Verification items for the finished model (mm, model axes). A direction names the side the tool comes from. Coordinates: 2 decimals unless noted, no trailing zeros. Write each loop counter-clockwise with the first axis right and the second up, starting at its lowest first coordinate (ties: lowest second). Pieces come first, ordered by that corner, then holes. Notation, with made-up numbers: (-14, 12.25) -> (44, 12.25) arc R27 ccw to (44, 51.25) -> close; hole circle Ø8 at (66, 1.5). An arc over 180 degrees is marked (long way). Write item = value, one per line. Start each with the question number.
(1) Section check B-B (y = -96.52). Record the cut outline in (x, z) (3 decimals), plus the area to 3 significant figures.
(2) Set-up check for faces 1 (the face through (-19, -469.9, -5)), 2 (the face through (180, 0, -5)), 3 (the face through (-19, -571.5, -5)), 4 (the face through (-11.6, -18.8, -4.9)), 5 (the face through (350.168, -500.631, -3.863)): record each of +Z, -Z, +X, -X, +Y, -Y from which the full face is reachable in a straight line by a thin tool's end or side.
(3) Gauge pin test, flat ends, axial feed: pin 1 Ø12 at (x, y) = (137, -469.5) entering from -Z; pin 2 Ø2 at (y, z) = (-77, -7) entering from -X. Record the tip position at first contact, or that the pin passes through.
(4) Section check D-D (y = -319). Record the cut outline in (x, z).
(5) Section check A-A (x = 342.9). Record the cut outline in (y, z), plus the area to 3 significant figures.
(6) Material ranges on probe 1 along Y at (x, z) = (342.9, -4.5); probe 2 along Z at (x, y) = (94.5, -353); probe 3 along X at (y, z) = (-174, -1.5), recorded low to high. Write a range as [from, to].
(7) Mould release check, pull along X, two halves, no side actions. Record for faces 6 (the face through (-19, -546.1, -5)), 7 (the face through (349.94, -99.44, -3.86)), 8 (the face through (-11.6, -126.8, -4.9)): released by +X, released by -X, zero draft, split by the parting line, or undercut.
(8) Section check C-C (x = 105.5). Record the cut outline in (y, z), plus the area to 3 significant figures.
```python
from build123d import *

# Parameters (mm, degrees)
BOSS_EXTRUDE1_DEPTH     = 609.6
SHELL1_T                = -7.62
SKETCH3_W               = 28.861952205
SKETCH3_H               = 274.814581436
CUT_EXTRUDE2_DEPTH      = 609.6
SKETCH4_W               = 397.1798
SKETCH4_H               = 244.7798
CUT_EXTRUDE3_DEPTH      = 609.6
SKETCH5_W               = 397.1798
SKETCH5_H               = 7.62
CUT_EXTRUDE4_DEPTH      = 609.6
BOSS_EXTRUDE4_START     = 25.4
BOSS_EXTRUDE4_DEPTH     = 25.4
LPATTERN2_COUNT         = 3
LPATTERN2_PITCH         = 50.8
LPATTERN3_COUNT         = 2
LPATTERN3_PITCH         = 508
LPATTERN6_COUNT         = 2
LPATTERN6_PITCH         = 457.2
LPATTERN7_COUNT         = 2
LPATTERN7_PITCH         = 406.4
CUT_EXTRUDE5_DEPTH      = 660.835961681
CUT_EXTRUDE5_DEPTH_BACK = 660.835961681
SKETCH11_R              = 4.445
CUT_EXTRUDE6_DEPTH      = 660.835961681
CUT_EXTRUDE6_DEPTH_BACK = 660.835961681
CUT_EXTRUDE7_DEPTH      = 681.722733812
CUT_EXTRUDE7_DEPTH_BACK = 681.722733812
CUT_EXTRUDE8_DEPTH      = 713.602768959
CUT_EXTRUDE8_DEPTH_BACK = 713.602768959
SKETCH16_R              = 7.62


with BuildPart() as part:
    # Sketch1 → Boss-Extrude1 (new body)
    with BuildSketch(Plane(origin=(0, 0, 0), x_dir=(1, 0, 0), z_dir=(0, 1, 0))):
        with BuildLine():
            Line((0, 0), (381, 0))
            ThreePointArc((381, 0), (392.440846298, 4.738953702), (397.1798, 16.1798))
            Line((397.1798, 16.1798), (397.1798, 244.7798))
            ThreePointArc((397.1798, 244.7798), (392.440846298, 256.220646298), (381, 260.9596))
            Line((381, 260.9596), (0, 260.9596))
            ThreePointArc((0, 260.9596), (-11.440846298, 256.220646298), (-16.1798, 244.7798))
            Line((-16.1798, 244.7798), (-16.1798, 16.1798))
            ThreePointArc((-16.1798, 16.1798), (-11.440846298, 4.738953702), (0, 0))
        make_face()
    extrude(amount=-BOSS_EXTRUDE1_DEPTH)

    # Shell1
    shell1_openings = [part.faces().sort_by_distance(p)[0] for p in [
        (190.5, 0, -130.4798),
    ]]
    offset(amount=SHELL1_T, openings=shell1_openings, kind=Kind.INTERSECTION)

    # Sketch3 → Cut-Extrude2 (cut)
    with BuildSketch(Plane(origin=(0, 0, 0), x_dir=(1, 0, 0), z_dir=(0, 1, 0))):
        with Locations((395.430976103, 137.407290718)):
            Rectangle(SKETCH3_W, SKETCH3_H)
    extrude(amount=-CUT_EXTRUDE2_DEPTH, mode=Mode.SUBTRACT)

    # Sketch4 → Cut-Extrude3 (cut)
    with BuildSketch(Plane(origin=(0, 0, 0), x_dir=(1, 0, 0), z_dir=(0, 1, 0))):
        with Locations((182.4101, 138.5697)):
            Rectangle(SKETCH4_W, SKETCH4_H)
    extrude(amount=-CUT_EXTRUDE3_DEPTH, mode=Mode.SUBTRACT)

    # Sketch5 → Cut-Extrude4 (cut)
    with BuildSketch(Plane(origin=(0, 0, -16.1798), x_dir=(-1, 0, 0), z_dir=(0, 0, -1))):
        with Locations((-182.4101, -605.79)):
            Rectangle(SKETCH5_W, SKETCH5_H)
    extrude(amount=-CUT_EXTRUDE4_DEPTH, mode=Mode.SUBTRACT)

    # Sketch8 → Boss-Extrude4 (add)
    with BuildSketch(Plane(origin=(0, -63.5, 0), x_dir=(1, 0, 0), z_dir=(0, 1, 0)).offset(BOSS_EXTRUDE4_START)):
        with BuildLine():
            Line((-16.1798, 16.1798), (-31.4198, 16.1798))
            Line((-31.4198, 16.1798), (-31.4198, 3.2512))
            ThreePointArc((-31.4198, 3.2512), (-30.467545567, 0.952254433), (-28.1686, 0))
            Line((-28.1686, 0), (0, 0))
            ThreePointArc((0, 0), (-11.440846298, 4.738953702), (-16.1798, 16.1798))
        make_face()
    boss_extrude4 = extrude(amount=-BOSS_EXTRUDE4_DEPTH)

    # LPattern2: Boss-Extrude4 ×3
    with Locations(*[(0, -i * LPATTERN2_PITCH, 0) for i in range(1, LPATTERN2_COUNT)]):
        add(boss_extrude4)

    # LPattern3: Boss-Extrude4 ×2
    with Locations(*[(0, -i * LPATTERN3_PITCH, 0) for i in range(1, LPATTERN3_COUNT)]):
        add(boss_extrude4)

    # LPattern6: Boss-Extrude4 ×2
    with Locations(*[(0, -i * LPATTERN6_PITCH, 0) for i in range(1, LPATTERN6_COUNT)]):
        add(boss_extrude4)

    # LPattern7: Boss-Extrude4 ×2
    with Locations(*[(0, -i * LPATTERN7_PITCH, 0) for i in range(1, LPATTERN7_COUNT)]):
        add(boss_extrude4)

    # Sketch11 → Cut-Extrude5 (cut, two sides: drawn at the far end of the back side and taken through both)
    with BuildSketch(Plane(origin=(0, -63.5, 0), x_dir=(1, 0, 0), z_dir=(0, 1, 0)).offset(-CUT_EXTRUDE5_DEPTH_BACK)):
        with Locations(Location((-22.7838, 8.5598, 0), (0, 0, 270))):
            Circle(SKETCH11_R)
    extrude(amount=CUT_EXTRUDE5_DEPTH + CUT_EXTRUDE5_DEPTH_BACK, mode=Mode.SUBTRACT)

    # Sketch14 → Cut-Extrude6 (cut, two sides: drawn at the far end of the back side and taken through both)
    with BuildSketch(Plane(origin=(0, -63.5, 0), x_dir=(1, 0, 0), z_dir=(0, 1, 0)).offset(-CUT_EXTRUDE6_DEPTH_BACK)):
        with BuildLine():
            Line((-23.2901518, 16.1798), (-23.2901518, 22.367061587))
            Line((-23.2901518, 22.367061587), (-43.448334217, 22.367061587))
            Line((-43.448334217, 22.367061587), (-43.448334217, 8.0501518))
            Line((-43.448334217, 8.0501518), (-31.4198, 8.0501518))
            ThreePointArc((-31.4198, 8.0501518), (-29.038681171, 13.798681171), (-23.2901518, 16.1798))
        make_face()
    extrude(amount=CUT_EXTRUDE6_DEPTH + CUT_EXTRUDE6_DEPTH_BACK, mode=Mode.SUBTRACT)

    # Sketch15 → Cut-Extrude7 (cut, two sides: drawn at the far end of the back side and taken through both)
    with BuildSketch(Plane(origin=(0, -38.1, 0), x_dir=(1, 0, 0), z_dir=(0, 1, 0)).offset(-CUT_EXTRUDE7_DEPTH_BACK)):
        with BuildLine():
            Line((-31.4198, 6.877959665), (-31.4198, 0))
            Line((-31.4198, 0), (-24.541840335, 0))
            ThreePointArc((-24.541840335, 0), (-29.405292255, 2.014507745), (-31.4198, 6.877959665))
        make_face()
    extrude(amount=CUT_EXTRUDE7_DEPTH + CUT_EXTRUDE7_DEPTH_BACK, mode=Mode.SUBTRACT)

    # Sketch16 → Cut-Extrude8 (cut, two sides: drawn at the far end of the back side and taken through both)
    with BuildSketch(Plane.XY.offset(-CUT_EXTRUDE8_DEPTH_BACK)):
        with Locations((342.9, -96.52)):
            Circle(SKETCH16_R)
        with Locations((342.9, -502.92)):
            Circle(SKETCH16_R)
    extrude(amount=CUT_EXTRUDE8_DEPTH + CUT_EXTRUDE8_DEPTH_BACK, mode=Mode.SUBTRACT)


solid = part.part
```
Response:
q1.outline = (-31.42, -8.05) arc R8.13 ccw to (-23.29, -16.18) -> (-8.56, -16.18) arc R8.56 cw to (0, -7.62) -> (335.28, -7.62) -> (335.28, 0) -> (-24.542, 0) arc R6.878 ccw to (-31.42, -6.878) -> close; (350.52, -7.62) -> (381, -7.62) -> (381, 0) -> (350.52, 0) -> close; hole circle Ø8.89 at (-22.784, -8.56)
q1.area = 3,150 mm2
q2.face_1 = +Z, -X
q2.face_2 = +Z, -Z, +X, -X, +Y
q2.face_3 = +Z, -X, -Y
q2.face_4 = +Z, -X, +Y
q2.face_5 = +Z, -Z
q3.pin_1 = -7.62
q3.pin_2 = -13.96
q4.outline = (-16.18, -16.18) -> (-8.56, -16.18) arc R8.56 cw to (0, -7.62) -> (381, -7.62) -> (381, 0) -> (0, 0) arc R16.18 ccw to start
q5.outline = (-601.98, -7.62) -> (-510.54, -7.62) -> (-510.54, 0) -> (-601.98, 0) -> close; (-495.3, -7.62) -> (-104.14, -7.62) -> (-104.14, 0) -> (-495.3, 0) -> close; (-88.9, -7.62) -> (0, -7.62) -> (0, 0) -> (-88.9, 0) -> close
q5.area = 4,350 mm2
q6.probe_1 = [-601.98, -510.54], [-495.3, -104.14], [-88.9, 0]
q6.probe_2 = [-7.62, 0]
q6.probe_3 = [-6.8, 381]
q7.face_6 = zero draft
q7.face_7 = undercut
q7.face_8 = released by -X
q8.outline = (-601.98, -7.62) -> (0, -7.62) -> (0, 0) -> (-601.98, 0) -> close
q8.area = 4,590 mm2
